Study the drawing (mm; zero at the part's minimum x, y, z) and answer. A direction names the side the tool comes from. Give positions to 0.01 mm unless a question says otherwise; leave off trailing zeros. Order: outer loops, then holes, each group sorted by start corner. A loop starts at its lowest first (then second) coordinate and runs counter-clockwise, first axis right, second up. Notation, with made-up numbers: (42, 63) - (77, 63) arc R20 ccw to (77, 87) - close; hole circle Ø3 at (37.5, -19.5). An arc over 180 degrees is marked (long way). Put each result on its own line as item: value.
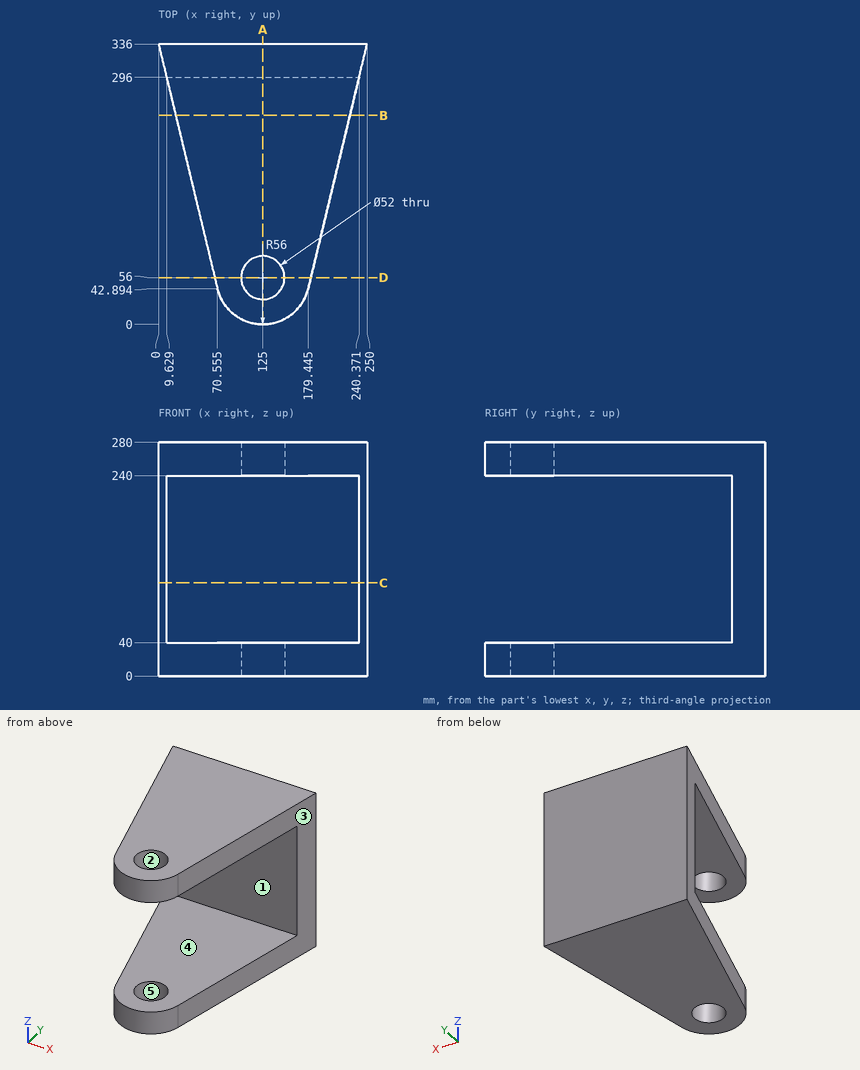
(1) Given pin 1 (4 mm diameter, centred on x = 89.5, y = 92.5, fed in from -Z), flat-ended and moving along its own axis, determine where the tip first touches the part or whether it passes through.
Geometry check:
pin 1: stops at z = 0
(2) Determine the mould class of the marked faces 3, 4 and 5 for opening direction Y: pulls with the +Y half, pulls with the -Y half, needs draft (parallel to the pull), parting line crosses it, or undercut.
Geometry check:
face 3: pulls with the -Y half
face 4: needs draft
face 5: undercut
(3) Section D-D, the plane y = 56 is taken. Write down the section's boundary in (x, z).
Geometry check:
outline: (67.4, 0) - (99, 0) - (99, 40) - (67.4, 40) - close; (67.4, 240) - (99, 240) - (99, 280) - (67.4, 280) - close; (151, 0) - (182.6, 0) - (182.6, 40) - (151, 40) - close; (151, 240) - (182.6, 240) - (182.6, 280) - (151, 280) - close
(4) Section A-A, the plane x = 125 is taken. Write down the section's boundary in (y, z), then the cut area to 3 significant figures.
Geometry check:
outline: (0, 0) - (30, 0) - (30, 40) - (0, 40) - close; (0, 240) - (30, 240) - (30, 280) - (0, 280) - close; (82, 0) - (336, 0) - (336, 280) - (82, 280) - (82, 240) - (296, 240) - (296, 40) - (82, 40) - close
area: 30,700 mm²
(5) A tool of negligible diameter and unlimited length cuts with its end or side. For the marked faces 1 and 2, from which of +Z, -Z, +X, -X, +Y, -Y can it reach the whole face along a straight path? Write none if from no direction.
Geometry check:
face 1: +X, -X, -Y
face 2: +Z, -Z
(6) Straight lines are drawn through the part: line 1 (Z direction, x = 158, y = 155.5); line 2 (Y direction, x = 125, z = 24); line 3 (Y direction, x = 62.5, z = 60.5). For each, find the intervals that lie inside material, in ascending order.
Geometry check:
line 1: z = 0 to 40, 240 to 280
line 2: y = 0 to 30, 82 to 336
line 3: y = 296 to 336
(7) Section C-C, the plane z = 111.5 is taken. Write down the section's boundary in (x, y).
Geometry check:
outline: (0, 336) - (9.63, 296) - (240.37, 296) - (250, 336) - close
(8) Section B-B, the plane y = 250.5 is taken. Write down the section's boundary in (x, z).
Geometry check:
outline: (20.58, 0) - (229.42, 0) - (229.42, 40) - (20.58, 40) - close; (20.58, 240) - (229.42, 240) - (229.42, 280) - (20.58, 280) - close
